Can you work these out from the model? Positions are in its coordinate system, mm. A direction names the side the tool comes from. Round coordinates to 2 decimals unless told otherwise and drop trailing zeros. Loops run counter-clockwise (first coordinate to the right, second up) from the corner with the lowest first, then second, coordinate; pieces in that order, holes last. Notation, with made-up numbers: (48, -21.75) -> (72, -21.75) arc R17 ccw to (72, -6.75) -> close; hole circle Ø7 at (64.5, 14). An arc over 180 degrees is marked (long way). Use a Markdown table: item, result.
Autodesk Inventor part; units mm, degrees
ref_plane "Arbeitsebene1" through (-41.75, -38.25, 1.6) normal (0, -1, 0) x (1, 0, 0)
ref_plane "YZ Plane" through (0, 0, 0) normal (1, 0, 0) x (0, 1, 0)
ref_plane "XZ Plane" through (0, 0, 0) normal (0, 1, 0) x (-1, 0, 0)
sketch "Skizze1" plane through (0, 0, 0) normal (0, 0, 1) x (1, 0, 0)
  line L0 (45.25, 50.25) -> (-45.25, 50.25)
  line L1 (-45.25, 50.25) -> (-45.25, -50.25)
  line L2 (-45.25, -50.25) -> (45.25, -50.25)
  line L3 (45.25, -50.25) -> (45.25, 50.25)
  line L4 (45.25, 50.25) -> (-45.25, -50.25) construction
  line L5 (-45.25, 50.25) -> (45.25, -50.25) construction
  point P0 (0, 0)
  dimension "d0" = 90.5
  dimension "d1" = 100.5
extrude "Extrusion1" add sketch "Skizze1" along normal blind 1.6
fillet "Rundung1" radius 5 4 edges at (45.25, 50.25, 0.8) (-45.25, 50.25, 0.8) (45.25, -50.25, 0.8) (-45.25, -50.25, 0.8)
sketch "Skizze2" plane through (0, 0, 0) normal (0, 0, -1) x (-1, 0, 0)
  line L0 (-5.75, -11.25) -> (0.75, -11.25)
  line L1 (0.75, -11.25) -> (0.75, -17.75)
  line L2 (0.75, -17.75) -> (-5.75, -17.75)
  line L3 (-5.75, -17.75) -> (-5.75, -11.25)
  line L4 (-5.75, -11.25) -> (0.75, -17.75) construction
  line L5 (0.75, -11.25) -> (-5.75, -17.75) construction
  line L6 (40.25, -50.25) -> (-40.25, -50.25)
  line L7 (-45.25, -45.25) -> (-45.25, 45.25)
  point P0 (0, 0)
  point P1 (-2.5, -14.5)
  point P2 (-2.5, -17.75)
  dimension "d5" = 32.5
  dimension "d6" = 39.5
  dimension "d7" = 6.5
  dimension "d8" = 6.5
extrude "Extrusion2" add sketch "Skizze2" along normal blind 5
fillet "Rundung2" radius 0.5 4 edges at (-0.75, -11.25, -2.5) (-0.75, -17.75, -2.5) (5.75, -17.75, -2.5) (5.75, -11.25, -2.5)
sketch "Skizze3" plane through (0, 0, 0) normal (0, 0, -1) x (-1, 0, 0)
  line L0 (38.25, -33.75) -> (45.25, -33.75)
  line L1 (45.25, -33.75) -> (45.25, -42.75)
  line L2 (45.25, -42.75) -> (38.25, -42.75)
  line L3 (38.25, -42.75) -> (38.25, -33.75)
  line L4 (38.25, -33.75) -> (45.25, -42.75) construction
  line L5 (45.25, -33.75) -> (38.25, -42.75) construction
  line L6 (40.25, -50.25) -> (-40.25, -50.25)
  line L7 (45.25, 45.25) -> (45.25, -45.25)
  point P0 (0, 0)
  point P1 (41.75, -38.25)
  dimension "d12" = 7.5
  dimension "d13" = 7
  dimension "d14" = 9
extrude "Extrusion3" add sketch "Skizze3" along normal blind 5
fillet "Rundung3" radius 2 2 edges at (-41.75, -33.75, -5) (-41.75, -42.75, -5)
sketch "Skizze4" plane through (0, 0, 1.6) normal (0, 0, 1) x (1, 0, 0)
  line L0 (39.25, 42.25) -> (45.25, 42.25)
  line L1 (45.25, 42.25) -> (45.25, 34.75)
  line L2 (45.25, 34.75) -> (39.25, 34.75)
  line L3 (39.25, 34.75) -> (39.25, 42.25)
  line L4 (39.25, 42.25) -> (45.25, 34.75) construction
  line L5 (45.25, 42.25) -> (39.25, 34.75) construction
  line L6 (45.25, -45.25) -> (45.25, 45.25)
  line L7 (-45.25, 45.25) -> (-45.25, -45.25)
  line L8 (40.25, 50.25) -> (-40.25, 50.25)
  line L9 (-43.25, 42.25) -> (-38.75, 42.25)
  line L10 (-38.75, 42.25) -> (-38.75, 33.25)
  line L11 (-38.75, 33.25) -> (-43.25, 33.25)
  line L12 (-43.25, 33.25) -> (-43.25, 42.25)
  line L13 (-43.25, 42.25) -> (-38.75, 33.25) construction
  line L14 (-38.75, 42.25) -> (-43.25, 33.25) construction
  point P0 (0, 0)
  point P1 (42.25, 38.5)
  point P2 (42.25, 42.25)
  point P3 (-41, 37.75)
  dimension "d19" = 8
  dimension "d20" = 7.5
  dimension "d21" = 6
  dimension "d22" = 8
  dimension "d23" = 9
  dimension "d24" = 4.5
  dimension "d25" = 2
extrude "Extrusion4" add sketch "Skizze4" along normal blind 4.5
sketch "Skizze5" plane through (-43.25, 33.25, 1.6) normal (-1, 0, 0) x (0, 0, 1)
  line L0 (1.5, 1.5) -> (3.5, 1.5)
  line L1 (3.5, 1.5) -> (3.5, 7.5)
  line L2 (3.5, 7.5) -> (1.5, 7.5)
  line L3 (1.5, 7.5) -> (1.5, 1.5)
  line L4 (1.5, 1.5) -> (3.5, 7.5) construction
  line L5 (3.5, 1.5) -> (1.5, 7.5) construction
  line L6 (0, 9) -> (4.5, 9)
  line L7 (4.5, 9) -> (4.5, 0)
  point P0 (-1.6, -33.25)
  point P1 (2.5, 4.5)
  dimension "d28" = 1.5
  dimension "d29" = 6
  dimension "d30" = 1
  dimension "d31" = 2
extrude "Extrusion5" add sketch "Skizze5" along normal blind 3
sketch "Skizze6" plane through (0, 0, 1.6) normal (0, 0, 1) x (1, 0, 0)
  line L0 (-41.75, 32.75) -> (41.75, 32.75)
  line L1 (41.75, 32.75) -> (41.75, -44.25)
  line L2 (41.75, -44.25) -> (-41.75, -44.25)
  line L3 (-41.75, -44.25) -> (-41.75, 32.75)
  line L4 (-41.75, 32.75) -> (41.75, -44.25) construction
  line L5 (41.75, 32.75) -> (-41.75, -44.25) construction
  line L6 (-40.25, -50.25) -> (40.25, -50.25)
  line L7 (-45.25, 45.25) -> (-45.25, -45.25)
  line L8 (45.25, -45.25) -> (45.25, 34.75)
  point P0 (0, 0)
  point P1 (0, -5.75)
  dimension "d34" = 6
  dimension "d35" = 3.5
  dimension "d36" = 3.5
  dimension "d37" = 77
extrude "Extrusion6" add sketch "Skizze6" along normal blind 15
ref_plane "Arbeitsebene1" through (-41.75, -38.25, 1.6) normal (0, -1, 0) x (1, 0, 0)
sketch "Skizze7" plane through (-41.75, -38.25, 1.6) normal (0, -1, 0) x (1, 0, 0)
  circle A0 centre (10.25, 10.4) radius 9
  circle A1 centre (31.25, 10.4) radius 9
  circle A2 centre (52.25, 10.4) radius 9
  circle A3 centre (73.25, 10.4) radius 9
  line L0 (1.5, -1.6) -> (82, -1.6)
  line L1 (10.25, 10.4) -> (114.75, 10.4) construction
  line L2 (0, 0) -> (83.5, 0) construction
  point P0 (41.75, -1.6)
  point P1 (62.5, 10.4)
  point P2 (41.75, 0)
  dimension "d41" = 18
  dimension "d42" = 18
  dimension "d43" = 18
  dimension "d44" = 18
  dimension "d45" = 21
  dimension "d46" = 21
  dimension "d47" = 21
  dimension "d49" = 31.5
  dimension "d50" = 21
extrude "Extrusion7" add sketch "Skizze7" against normal blind 65
sketch "Skizze8" plane through (0, 0, 1.6) normal (0, 0, 1) x (1, 0, 0)
  line L0 (-37.75, 47.25) -> (37.75, 47.25)
  line L1 (37.75, 47.25) -> (37.75, -47.75)
  line L2 (37.75, -47.75) -> (-37.75, -47.75)
  line L3 (-37.75, -47.75) -> (-37.75, 47.25)
  line L4 (41.75, 32.75) -> (-41.75, 32.75)
  line L5 (40.25, 50.25) -> (-40.25, 50.25)
  point P0 (0, 0)
  point P1 (0, 32.75)
  point P2 (0, 47.25)
  dimension "d53" = 95
  dimension "d54" = 75.5
  dimension "d55" = 0
  dimension "d56" = 3
hole "Bohrung1" at (-37.75, 47.25, 1.6) at (37.75, 47.25, 1.6) at (-37.75, -47.75, 1.6) at (37.75, -47.75, 1.6) direction (0, 0, -1) diameter 3 depth 1.6
properties part number "010_Battery_2Cell"
1. I want a section at D-D (z = 8). Please give me the cut outline in (x, y), plus the area to 3 significant figures.
Answer sheet:
| item | result |
|---|---|
| outline | (-41.75, -44.25) -> (41.75, -44.25) -> (41.75, 32.75) -> (-41.75, 32.75) -> close |
| area | 6,430 mm² |
2. I want a section at B-B (y = 8). Please give me the cut outline in (x, z), plus the area to 3 significant figures.
Answer sheet:
| item | result |
|---|---|
| outline | (-45.25, 0) -> (45.25, 0) -> (45.25, 1.6) -> (41.75, 1.6) -> (41.75, 16.6) -> (39.24, 16.6) arc R9 ccw to (23.76, 16.6) -> (18.24, 16.6) arc R9 ccw to (2.76, 16.6) -> (-2.76, 16.6) arc R9 ccw to (-18.24, 16.6) -> (-23.76, 16.6) arc R9 ccw to (-39.24, 16.6) -> (-41.75, 16.6) -> (-41.75, 1.6) -> (-45.25, 1.6) -> close |
| area | 1,590 mm² |
3. I need wall thicknesses on line 1 (Y direction, x = -37.75, z = 0.4); line 2 (X direction, y = 47.25, z = 0.55); line 3 (X direction, y = -7, z = 20.25). Which ranges of each line are inside material? Lowest first, please.
Answer sheet:
| item | result |
|---|---|
| line 1 | y = -50.25 to -49.25, -46.25 to 45.75, 48.75 to 50.25 |
| line 2 | x = -44.83 to -39.25, -36.25 to 36.25, 39.25 to 44.83 |
| line 3 | x = -35.1 to -27.9, -14.1 to -6.9, 6.9 to 14.1, 27.9 to 35.1 |
4. I want a section at A-A (x = 37.75). Please give me the cut outline in (y, z), plus the area to 3 significant figures.
Answer sheet:
| item | result |
|---|---|
| outline | (-50.25, 0) -> (-49.25, 0) -> (-49.25, 1.6) -> (-50.25, 1.6) -> close; (-46.25, 0) -> (45.75, 0) -> (45.75, 1.6) -> (32.75, 1.6) -> (32.75, 16.6) -> (26.75, 16.6) -> (26.75, 18.48) -> (-38.25, 18.48) -> (-38.25, 16.6) -> (-44.25, 16.6) -> (-44.25, 1.6) -> (-46.25, 1.6) -> close; (48.75, 0) -> (50.25, 0) -> (50.25, 1.6) -> (48.75, 1.6) -> close |
| area | 1,430 mm² |
5. Which directions (+Z, -Z, +X, -X, +Y, -Y) give clear straight access to the entire face, cutting with the end or side of a thin tool? Please do faces 4 (the flat face through (39.25, 38, 4)), 5 (the flat face through (-1, -5, 16.6)), 6 (the flat face through (-41, 38, 6.1)).
Answer sheet:
| item | result |
|---|---|
| face 4 | +Z, +Y |
| face 5 | +Z |
| face 6 | +Z, +X, -X, +Y |
6. If we mould it in two halves opening along Y, with no side actions, what happens to faces 1 (the cylindrical face through (43.82, 48.75, 0.81)), 2 (the cylindrical face through (-36.84, -46.56, 0.79)), 3 (the flat face through (-11, -38.25, 18))? For each: +Y half, -Y half, draft (parallel to the pull), parting line (faces both ways), or undercut.
Answer sheet:
| item | result |
|---|---|
| face 1 | +Y half |
| face 2 | undercut |
| face 3 | -Y half |
7. Will these pins go through, and if not, where does the flat tip stop? pin 1 Ø0.6 at (x, z) = (-45.5, 4.5) entering from +Y; pin 2 Ø3.5 at (y, z) = (39, 3) entering from -X; pin 3 Ø3.5 at (x, z) = (-12, 18.5) entering from -Y; pin 4 Ø3 at (y, z) = (-34, 11.5) entering from +X.
Answer sheet:
| item | result |
|---|---|
| pin 1 | stops at y = 40.75 |
| pin 2 | stops at x = -46.25 |
| pin 3 | stops at y = -38.25 |
| pin 4 | stops at x = 41.75 |
8. I want a section at C-C (y = 47.25). Please give me the cut outline in (x, z).
Answer sheet:
| item | result |
|---|---|
| outline | (-44.83, 0) -> (-39.25, 0) -> (-39.25, 1.6) -> (-44.83, 1.6) -> close; (-36.25, 0) -> (36.25, 0) -> (36.25, 1.6) -> (-36.25, 1.6) -> close; (39.25, 0) -> (44.83, 0) -> (44.83, 1.6) -> (39.25, 1.6) -> close |
